Part model, mm, in its own coordinate system. Give positions to 0.01 mm unless a question says otherwise; leave off trailing zeros. Order: outer loops, then holes, each group sorted by start corner. A loop starts at its lowest first (then second) coordinate and runs counter-clockwise, first axis right, second up. Notation, with made-up numbers: (72, 16.25) - (99, 16.25) arc R21 cw to (99, 50.25) - close; hole circle Ø9 at (3, 50.5). An arc over 180 degrees is marked (long way). Use one line per item in the form item = value. Start each with the question number.
1. Band-saw the part on A-A, the plane x = 112.58. List the corners of the cut face in (y, z).
2. Drill centre line: line 1 (Z direction, x = 112.58, y = 1.1). Where is it in solid material? Low to high.
3. Pin check, flat tips, straight feed: P1, Ø1.4, axis at y = 1.5, z = -23.5, coming from the +X side; P2, Ø1.4, axis at x = 186, y = 1.5, coming from the -Z side. Stop position of each tip, or through.
4. Band-saw the part on B-B, the plane z = -419.6. List the corners of the cut face in (x, y), plus the area to 3 significant figures.
from build123d import *

# Parameters (mm, degrees)
SKETCH1_W           = 190.5
SKETCH1_H           = 609.6
BOSS_EXTRUDE1_DEPTH = 2.778125
SKETCH2_W           = 190.5
SKETCH2_H           = 17.78
CUT_EXTRUDE1_DEPTH  = 3.778125
SKETCH3_W           = 17.78
SKETCH3_H           = 574.04
CUT_EXTRUDE2_DEPTH  = 3.778125
SKETCH4_W           = 10.16
SKETCH4_H           = 10.16
CUT_EXTRUDE3_DEPTH  = 3.778125
FILLET1_R           = 2.54
SKETCH5_R           = 9
CUT_EXTRUDE4_DEPTH  = 3.778125


with BuildPart() as part:
    # Sketch1 → Boss-Extrude1 (new body)
    with BuildSketch(Plane(origin=(0, 0, 0), x_dir=(1, 0, 0), z_dir=(0, 1, 0))):
        with Locations((95.25, 304.8)):
            Rectangle(SKETCH1_W, SKETCH1_H)
    extrude(amount=BOSS_EXTRUDE1_DEPTH)

    # Sketch2 → Cut-Extrude1 (cut, through all)
    with BuildSketch(Plane(origin=(0, 2.778125, 0), x_dir=(1, 0, 0), z_dir=(0, 1, 0))):
        with Locations((95.25, 8.89)):
            Rectangle(SKETCH2_W, SKETCH2_H)
        with Locations((95.25, 600.71)):
            Rectangle(SKETCH2_W, SKETCH2_H)
    extrude(amount=-CUT_EXTRUDE1_DEPTH, mode=Mode.SUBTRACT)

    # Sketch3 → Cut-Extrude2 (cut, through all)
    with BuildSketch(Plane(origin=(0, 2.778125, 0), x_dir=(1, 0, 0), z_dir=(0, 1, 0))):
        with Locations((8.89, 304.8)):
            Rectangle(SKETCH3_W, SKETCH3_H)
    extrude(amount=-CUT_EXTRUDE2_DEPTH, mode=Mode.SUBTRACT)

    # Sketch4 → Cut-Extrude3 (cut, through all)
    with BuildSketch(Plane(origin=(0, 2.778125, 0), x_dir=(1, 0, 0), z_dir=(0, 1, 0))):
        with Locations((185.42, 586.74)):
            Rectangle(SKETCH4_W, SKETCH4_H)
        with Locations((185.42, 22.86)):
            Rectangle(SKETCH4_W, SKETCH4_H)
    extrude(amount=-CUT_EXTRUDE3_DEPTH, mode=Mode.SUBTRACT)

    # Fillet1
    fillet1_edges = [part.edges().sort_by_distance(p)[0] for p in [
        (17.78, 1.3890625, -591.82),
        (17.78, 1.3890625, -17.78),
        (190.5, 1.3890625, -581.66),
        (180.34, 1.3890625, -581.66),
        (180.34, 1.3890625, -591.82),
        (190.5, 1.3890625, -27.94),
        (180.34, 1.3890625, -17.78),
        (180.34, 1.3890625, -27.94),
    ]]
    fillet(fillet1_edges, radius=FILLET1_R)

    # Sketch5 → Cut-Extrude4 (cut, through all)
    with BuildSketch(Plane.XZ):
        with Locations((112.58, -419.599999967)):
            Circle(SKETCH5_R)
    extrude(amount=-CUT_EXTRUDE4_DEPTH, mode=Mode.SUBTRACT)


solid = part.part
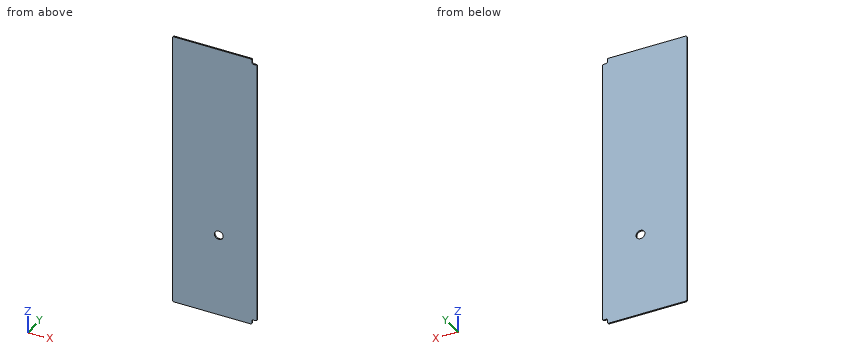
From the geometry:
q1.outline = (0, -591.82) - (2.78, -591.82) - (2.78, -428.6) - (0, -428.6) - close; (0, -410.6) - (2.78, -410.6) - (2.78, -17.78) - (0, -17.78) - close
q2.line_1 = -591.82 to -428.6, -410.6 to -17.78
q3.P1 = 180.34
q3.P2 = -581.66
q4.outline = (17.78, 0) - (103.58, 0) - (103.58, 2.78) - (17.78, 2.78) - close; (121.58, 0) - (190.5, 0) - (190.5, 2.78) - (121.58, 2.78) - close
q4.area = 430 mm²
